from build123d import *

# Parameters (mm, degrees)
F0_R          = 15.24
F0_R_2        = 12.7
F1_DEPTH      = 157.48
F0_R_3        = 19.05
F2_DEPTH      = 2.54
F3_R          = 19.05
F3_R_2        = 15.24
F4_DEPTH      = 2.54
F6_R          = 8.89
F6_R_2        = 6.35
F7_DEPTH      = 25.4
F7_DEPTH_BACK = 12.7
F8_R          = 12.7
F8_R_2        = 8.89
F9_DEPTH      = 2.54
F10_DEPTH     = 101.6
F8_R_3        = 6.35
F11_DEPTH     = 38.1


with BuildPart() as f1:
    # F0 (on Front) → F1 (new body)
    with BuildSketch(Plane.XZ):
        Circle(F0_R)
        Circle(F0_R_2, mode=Mode.SUBTRACT)
    extrude(amount=F1_DEPTH)

    # F0 (on Front) → F2 (join)
    with BuildSketch(Plane.XZ):
        Circle(F0_R_3)
        Circle(F0_R, mode=Mode.SUBTRACT)
    extrude(amount=F2_DEPTH)

    # F3 (on face) → F4 (join)
    with BuildSketch(Plane.XZ.offset(157.48)):
        Circle(F3_R)
        Circle(F3_R_2, mode=Mode.SUBTRACT)
    extrude(amount=-F4_DEPTH)

    # F6 (on offset) → F7 (join, two sides)
    with BuildSketch(Plane.XY.offset(25.4)) as f7_sk:
        with Locations((0, -78.74)):
            Circle(F6_R)
        with Locations((0, -78.74)):
            Circle(F6_R_2, mode=Mode.SUBTRACT)
    extrude(amount=-F7_DEPTH)
    extrude(f7_sk.sketch, amount=F7_DEPTH_BACK)

    # F8 (on face) → F9 (join)
    with BuildSketch(Plane.XY.offset(38.1)):
        with Locations((0, -78.74)):
            Circle(F8_R)
        with Locations((0, -78.74)):
            Circle(F8_R_2, mode=Mode.SUBTRACT)
    extrude(amount=-F9_DEPTH)

    # F0 (on Front) → F10 (cut)
    with BuildSketch(Plane.XZ):
        Circle(F0_R_2)
    extrude(amount=F10_DEPTH, mode=Mode.SUBTRACT)

    # F8 (on face) → F11 (cut)
    with BuildSketch(Plane.XY.offset(38.1)):
        with Locations((0, -78.74)):
            Circle(F8_R_3)
    extrude(amount=-F11_DEPTH, mode=Mode.SUBTRACT)


solid = f1.part
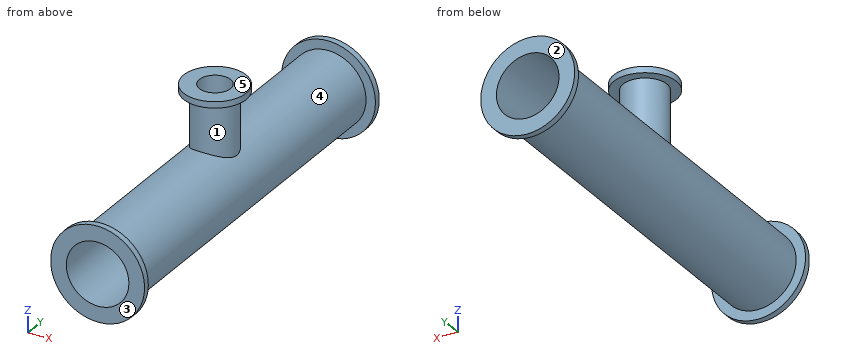
CAD build for the part. Positions are in the model's coordinates, mm. Face numbers are marked on the shaded views. A direction names the side the tool comes from. Give positions to 0.01 mm unless a question says otherwise; leave off trailing zeros. Loops run counter-clockwise (first coordinate to the right, second up) from the corner with the lowest first, then second, coordinate; pieces in that order, holes last. Notation, with made-up numbers: M 46.5,-39 L 50.5,-39 A24 ccw 50.5,-7 Z; hole C -23.75,21.25 d4. An arc over 180 degrees is marked long. Answer in a Markdown table with one row per item. Add a question column.
Item 1: Band-saw the part on D-D on z = 17. Give the cut face in (x, y), then the cut area to 3 significant figures.
Item 2: Tool access for the marked faces 1 and 2: list every direction of +Z, -Z, +X, -X, +Y, -Y with a clear straight run to the whole face (end or side of a thin tool).
Item 3: Band-saw the part on A-A on x = 0. Give the cut face in (y, z).
Item 4: Mould opens along Y. For the marked faces 3, 4 and 5 say: +Y half, -Y half, draft (parallel to the pull), parting line (faces both ways), or undercut.
Item 5: Drop flat-ended pins along their axis: P1, Ø6, axis at x = -5.5, y = -134, coming from the +Z side; P2, Ø12, axis at y = -35, z = 0, coming from the -X side; P3, Ø4, axis at x = 12, y = -132.5, coming from the +Z side; P4, Ø20.5, axis at x = 0, z = 0, coming from the -Y side. Give the stop position or say it passes through.
Item 6: Band-saw the part on C-C on y = -78.74. Give the cut face in (x, z), then the cut area to 3 significant figures.
Item 7: Probe probe 1 along Y at (x, z) = (12, -12.5); probe 2 along X at (y, z) = (-78.74, 23); probe 3 along Z at (x, y) = (0, -128). List the from-to ranges inside material, lowest first.
Item 8: Band-saw the part on B-B on z = -2. Give the cut face in (x, y), then the cut area to 3 significant figures.
Reply:
| question | item | result |
|---|---|---|
| 1 | outline | C 0,-78.74 d17.78; M -8.6,-157.48 L 8.6,-157.48 L 8.6,-154.94 L -8.6,-154.94 Z; M -8.6,-2.54 L 8.6,-2.54 L 8.6,0 L -8.6,0 Z; hole C 0,-78.74 d12.7 |
| 1 | area | 209 mm^2 |
| 2 | face 1 | none |
| 2 | face 2 | +Z, -Z, +X, -X, +Y |
| 3 | outline | M -157.48,-19.05 L -154.94,-19.05 L -154.94,-15.24 L -2.54,-15.24 L -2.54,-19.05 L 0,-19.05 L 0,-12.7 L -157.48,-12.7 Z; M -157.48,12.7 L -85.09,12.7 L -85.09,38.1 L -91.44,38.1 L -91.44,35.56 L -87.63,35.56 L -87.63,15.24 L -154.94,15.24 L -154.94,19.05 L -157.48,19.05 Z; M -72.39,12.7 L 0,12.7 L 0,19.05 L -2.54,19.05 L -2.54,15.24 L -69.85,15.24 L -69.85,35.56 L -66.04,35.56 L -66.04,38.1 L -72.39,38.1 Z |
| 4 | face 3 | -Y half |
| 4 | face 4 | undercut |
| 4 | face 5 | draft |
| 5 | P1 | stops at z = 15.03 |
| 5 | P2 | stops at x = -15.24 |
| 5 | P3 | stops at z = 11.5 |
| 5 | P4 | passes through |
| 6 | outline | M -12.7,35.56 L -8.89,35.56 L -8.89,12.38 A15.24 ccw long 8.89,12.38 L 8.89,35.56 L 12.7,35.56 L 12.7,38.1 L 6.35,38.1 L 6.35,11 A12.7 cw long -6.35,11 L -6.35,38.1 L -12.7,38.1 Z |
| 6 | area | 335 mm^2 |
| 7 | probe 1 | y = -157.48 to -154.94, -2.54 to 0 |
| 7 | probe 2 | x = -8.89 to -6.35, 6.35 to 8.89 |
| 7 | probe 3 | z = -15.24 to -12.7, 12.7 to 15.24 |
| 8 | outline | M -18.94,-157.48 L -12.54,-157.48 L -12.54,0 L -18.94,0 L -18.94,-2.54 L -15.11,-2.54 L -15.11,-154.94 L -18.94,-154.94 Z; M 12.54,-157.48 L 18.94,-157.48 L 18.94,-154.94 L 15.11,-154.94 L 15.11,-2.54 L 18.94,-2.54 L 18.94,0 L 12.54,0 Z |
| 8 | area | 847 mm^2 |
